Design review of the part built by this model. Coordinates are the model's own, in mm. A direction names the side the tool comes from. Coordinates: 2 decimals unless noted, no trailing zeros. Write each loop counter-clockwise with the first axis right and the second up, starting at its lowest first coordinate (ties: lowest second). Pieces come first, ordered by that corner, then holes. Notation, with made-up numbers: (-24, 45) - (16, 45) arc R6 ccw to (16, 50) - close; hole circle Ø5 at (32.25, 44). An arc over 180 degrees is marked (long way). One line per item, written item: value.
from build123d import *

# Parameters (mm, degrees)
SKETCH_1_W          = 14
SKETCH_1_H          = 28
EXTRUDE_1_DEPTH     = 2
SKETCH_2_R          = 1.5
CUT_EXTRUDE_1_DEPTH = 2
SKETCH_3_W          = 14
SKETCH_3_H          = 2
EXTRUDE_2_DEPTH     = 7
FILLET_1_R          = 6
SKETCH_4_R          = 1.5
CUT_EXTRUDE_2_DEPTH = 15


with BuildPart() as part:
    # Эскиз1 → Бобышка-Вытянуть1 (new body)
    with BuildSketch(Plane.XZ):
        with Locations((7, -14)):
            Rectangle(SKETCH_1_W, SKETCH_1_H)
    extrude(amount=EXTRUDE_1_DEPTH)

    # Эскиз2 → Вырез-Вытянуть1 (cut)
    with BuildSketch(Plane.XZ.offset(2)):
        with Locations(Location((7, -5, 0), (0, 0, 270))):
            Circle(SKETCH_2_R)
        with Locations(Location((7, -23, 0), (0, 0, 270))):
            Circle(SKETCH_2_R)
    extrude(amount=-CUT_EXTRUDE_1_DEPTH, mode=Mode.SUBTRACT)

    # Эскиз3 → Бобышка-Вытянуть2 (add)
    with BuildSketch(Plane(origin=(0, 0, 0), x_dir=(1, 0, 0), z_dir=(0, 1, 0))):
        with Locations((7, 17)):
            Rectangle(SKETCH_3_W, SKETCH_3_H)
    extrude(amount=EXTRUDE_2_DEPTH)

    # Скругление1
    fillet_1_edges = [part.edges().sort_by_distance(p)[0] for p in [
        (0, -1, 0),
        (14, -1, 0),
        (14, -1, -28),
        (0, -1, -28),
    ]]
    fillet(fillet_1_edges, radius=FILLET_1_R)

    # Эскиз4 → Вырез-Вытянуть2 (cut)
    with BuildSketch(Plane(origin=(0, 0, -18), x_dir=(-1, 0, 0), z_dir=(0, 0, -1))):
        with Locations((-11, 4)):
            Circle(SKETCH_4_R)
        with Locations((-3, 4)):
            Circle(SKETCH_4_R)
    extrude(amount=-CUT_EXTRUDE_2_DEPTH, mode=Mode.SUBTRACT)


solid = part.part
1. Wall thickness on line 1 along Y through (x, z) = (11, -16.55); line 2 along Z through (x, y) = (1.5, 1); line 3 along Y through (x, z) = (2.5, -14.75): over which ranges is each line inside the solid? List them lowest first.
Answer block:
line 1: y = -2 to 2.5, 5.5 to 7
line 2: z = -18 to -16
line 3: y = -2 to 0
2. Consider section A-A, the plane x = 7. Write out the cut boundary in (y, z).
Answer block:
outline: (-2, -28) - (0, -28) - (0, -24.5) - (-2, -24.5) - close; (-2, -21.5) - (0, -21.5) - (0, -18) - (7, -18) - (7, -16) - (0, -16) - (0, -6.5) - (-2, -6.5) - close; (-2, -3.5) - (0, -3.5) - (0, 0) - (-2, 0) - close
3. Mouldability with a two-part tool opening along Y and no side actions: class faces 1 (the face through (7, 7, -17)), 2 (the face through (0, -0.5, -15.2)), 3 (the face through (1.57, 4.45, -17.01)) as released by +Y, released by -Y, zero draft, split by the parting line, or undercut.
Answer block:
face 1: released by +Y
face 2: zero draft
face 3: undercut
4. Consider section C-C, the plane y = 4. Write out the cut boundary in (x, z).
Answer block:
outline: (0, -18) - (1.5, -18) - (1.5, -16) - (0, -16) - close; (4.5, -18) - (9.5, -18) - (9.5, -16) - (4.5, -16) - close; (12.5, -18) - (14, -18) - (14, -16) - (12.5, -16) - close
5. Consider section B-B, the plane y = -1. Write out the cut boundary in (x, z).
Answer block:
outline: (0, -22) arc R6 ccw to (6, -28) - (8, -28) arc R6 ccw to (14, -22) - (14, -6) arc R6 ccw to (8, 0) - (6, 0) arc R6 ccw to (0, -6) - close; hole circle Ø3 at (7, -23); hole circle Ø3 at (7, -5)
6. For faces 4 (the face through (7, 0, -8)), 5 (the face through (1.711, -1.014, -26.196)), 6 (the face through (5, 0, -23)), list the 3-axis set-ups (+Z, -Z, +X, -X, +Y, -Y) from which the entire face can be reached by the end or side of a thin tool; tool diameter is ignored.
Answer block:
face 4: +Z, +X, -X, +Y
face 5: -Z, -X, +Y, -Y
face 6: -Z, +X, -X, +Y
7. Insertion check: pin 1 Ø1.5 at (x, z) = (4.5, -15) entering from +Y; pin 2 Ø8 at (x, z) = (3, -20) entering from +Y; pin 3 Ø1.5 at (x, y) = (2, 5.5) entering from -Z. Each pin has a flat end and moves straight along its axis. Give the tip position at first contact, or say it passes through.
Answer block:
pin 1: stops at y = 0
pin 2: stops at y = 7
pin 3: stops at z = -18
8. Consider section D-D, the plane x = 2. Write out the cut boundary in (y, z), then the cut area to 3 significant figures.
Answer block:
outline: (-2, -26.47) - (0, -26.47) - (0, -18) - (2.88, -18) - (2.88, -16) - (0, -16) - (0, -1.53) - (-2, -1.53) - close; (5.12, -18) - (7, -18) - (7, -16) - (5.12, -16) - close
area: 59.4 mm^2
